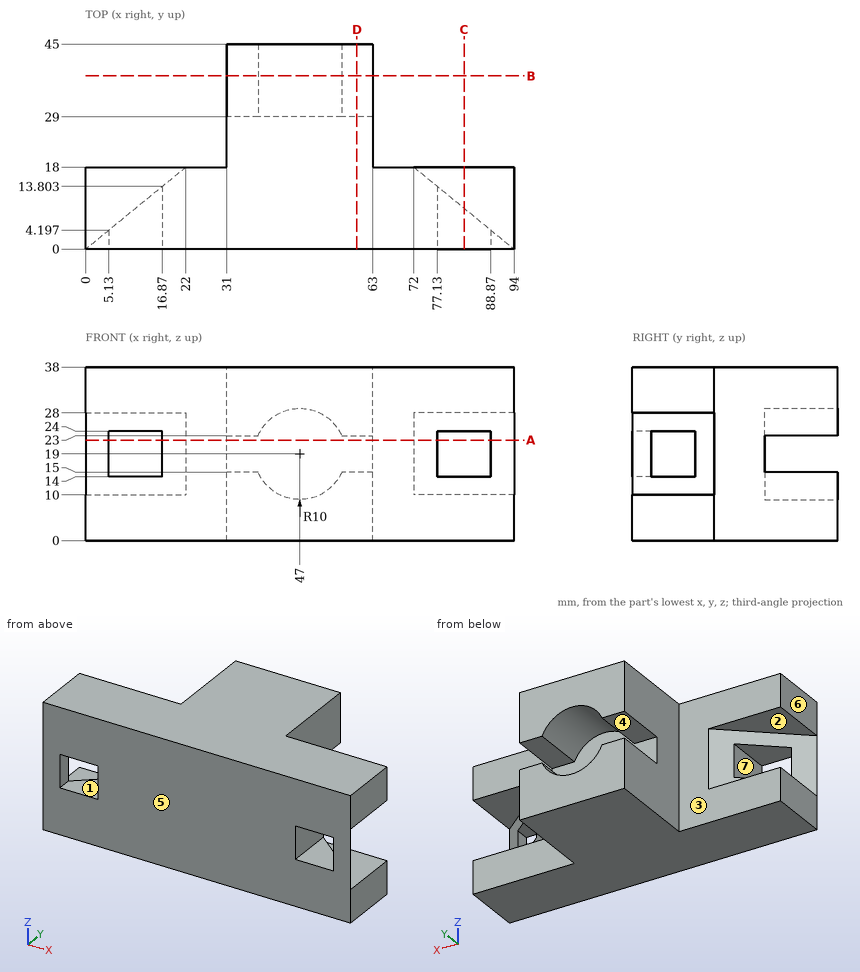
Input: dimensioned drawing with shaded views. Units: mm. Origin: part minimum x, y, z. A direction names the side the tool comes from. Coordinates: 2 decimals unless noted, no trailing zeros. Loops run counter-clockwise (first coordinate to the right, second up) from the corner with the lowest first, then second, coordinate; pieces in that order, holes last. Notation, with made-up numbers: M 64,80.25 L 101,80.25 A27 ccw 101,115.25 Z; hole C -1.75,-24.5 d7. An arc over 180 degrees is marked long. Use a Markdown table: item, result. Add a question column.
1) Draft query along X for the marked faces 5, 6 and 7. Return one class per face: +X half, -X half, draft (parallel to the pull), parting line (faces both ways), or undercut.
2) Line query: L1, parallel to Z at x = 85.5, y = 14; L2, parallel to X at y = 7, z = 22.5; L3, parallel to X at y = 40, z = 35.5. Output: solid intervals per line, ascending. Write a range as from..to.
3) Section D-D, the plane x = 59.5. Return the cut outline in (y, z), plus the area to 3 significant figures.
4) Set-up query: the marked faces 1, 2, 3 and 4. Return all of +Z, -Z, +X, -X, +Y, -Y with unobstructed straight access to the full face (end or side cutting, diameter ignored); none if empty.
5) Section C-C, the plane x = 83. Return the cut outline in (y, z), plus the area to 3 significant figures.
6) Pin query (flat end, axial travel): P1, Ø5.5, axis at x = 84, y = 5.5, coming from the -Z side; P2, Ø1.3, axis at y = 3, z = 19, coming from the -X side; P3, Ø1.5, axis at y = 13.5, z = 11.5, coming from the -X side; P4, Ø2, axis at y = 2, z = 20, coming from the +X side. Return the tip coordinate at first contact, or that it passes through.
7) Section B-B, the plane y = 38. Return the cut outline in (x, z) (1 decimal).
8) Section A-A, the plane z = 22. Return the cut outline in (x, y).
Answer below:
| question | item | result |
|---|---|---|
| 1 | face 5 | draft |
| 1 | face 6 | -X half |
| 1 | face 7 | undercut |
| 2 | L1 | 0..10, 28..38 |
| 2 | L2 | 16.87..77.13 |
| 2 | L3 | 31..63 |
| 3 | outline | M 0,0 L 45,0 L 45,15 L 29,15 L 29,23 L 45,23 L 45,38 L 0,38 Z |
| 3 | area | 1,580 mm2 |
| 4 | face 1 | +Y, -Y |
| 4 | face 2 | -X, +Y |
| 4 | face 3 | +Z, -Z, -X, +Y |
| 4 | face 4 | +X, -X, +Y |
| 5 | outline | M 0,0 L 18,0 L 18,10 L 9,10 L 9,14 L 0,14 Z; M 0,24 L 9,24 L 9,28 L 18,28 L 18,38 L 0,38 Z |
| 5 | area | 432 mm2 |
| 6 | P1 | z = 0 |
| 6 | P2 | x = 2.87 |
| 6 | P3 | x = 15.58 |
| 6 | P4 | x = 92.78 |
| 7 | outline | M 31,0 L 63,0 L 63,15 L 56.2,15 A10 cw 37.8,15 L 31,15 Z; M 31,23 L 37.8,23 A10 cw 56.2,23 L 63,23 L 63,38 L 31,38 Z |
| 8 | outline | M 0,0 L 5.13,0 L 5.13,4.2 Z; M 16.87,0 L 77.13,0 L 77.13,13.8 L 72,18 L 63,18 L 63,29 L 31,29 L 31,18 L 22,18 L 16.87,13.8 Z; M 88.87,0 L 94,0 L 88.87,4.2 Z |
